For this review, take the finished solid that the model builds, in its own axes (mm). A direction names the side the tool comes from. Coordinates: 2 decimals unless noted, no trailing zeros. Loops run counter-clockwise (first coordinate to the right, second up) from the corner with the lowest first, then second, coordinate; pieces in that order, holes last. Notation, with made-up numbers: M 22.25,81 L 56.25,81 A16 ccw 56.25,100 Z; hole C 23,23.25 d11. An arc over 180 degrees is marked long. Use one line per item in the form item = value.
Autodesk Inventor part; units mm, degrees
ref_plane "YZ Plane" through (0, 0, 0) normal (1, 0, 0) x (0, 1, 0)
ref_plane "XZ Plane" through (0, 0, 0) normal (0, 1, 0) x (-1, 0, 0)
ref_plane "XY Plane" through (0, 0, 0) normal (0, 0, 1) x (1, 0, 0)
sketch "Sketch1" plane through (0, 0, 0) normal (0, 0, 1) x (1, 0, 0)
  arc A0 (18.3475, -1.5748) -> (17.9494, -4.1148) centre (0, 0) ccw
  line L0 (-16.7386, -24.5618) -> (16.7386, -24.5618)
  line L1 (16.7386, -24.5618) -> (16.7386, -12.6068)
  line L2 (-16.7386, -12.6068) -> (-16.7386, -24.5618)
  line L3 (-20.955, 0) -> (-20.955, 20.955) construction
  line L4 (-20.955, 20.955) -> (25.273, 20.955) construction
  line L5 (16.7386, -24.5618) -> (25.273, -24.5618) construction
  line L6 (25.273, -24.5618) -> (25.273, -9.9568) construction
  line L7 (25.273, -9.9568) -> (21.0058, -9.9568) construction
  line L8 (25.273, -9.9568) -> (25.273, 2.1082) construction
  line L9 (25.273, 2.1082) -> (16.2735, 13.2017)
  line L10 (25.273, 2.1082) -> (25.273, -1.5748) construction
  line L11 (25.273, -1.5748) -> (18.3475, -1.5748)
  line L12 (25.273, 2.1082) -> (25.273, -1.5748)
  line L13 (25.273, -1.5748) -> (25.273, -4.1148) construction
  line L14 (25.273, -4.1148) -> (25.273, -9.9568)
  line L15 (25.273, -9.9568) -> (18.4384, -9.9568)
  line L16 (25.273, -4.1148) -> (17.9494, -4.1148)
  arc A1 (16.2735, 13.2017) -> (-16.7386, -12.6068) centre (0, 0) ccw
  arc A2 (16.7386, -12.6068) -> (18.4384, -9.9568) centre (0, 0) ccw
  dimension "d0" = 36.83
extrude "Extrusion1" add sketch "Sketch1" along normal blind 9.525
sketch "Sketch2" plane through (-16.7386, -24.5618, 0) normal (0, -1, 0) x (1, 0, 0)
  line L0 (0, 9.525) -> (33.4772, 9.525)
  line L1 (16.7386, 0) -> (16.7386, 9.525) construction
  line L2 (30.2133, 4.7625) -> (3.2639, 4.7625) construction
  circle A0 centre (3.2639, 4.7625) radius 1.7526
  circle A1 centre (30.2133, 4.7625) radius 1.7526
  dimension "d12" = 26.9494
  dimension "d13" = 3.5052
  dimension "d14" = 3.5052
extrude "Extrusion2" cut sketch "Sketch2" against normal blind 9.525
thread "Thread1"
thread "Thread2"
sketch "Sketch3" plane through (18.4384, -9.9568, 0) normal (0, -1, 0) x (1, 0, 0)
  line L0 (6.8346, 0) -> (6.8346, 9.525)
  line L1 (0, 0) -> (0, 9.525)
  line L2 (6.8346, 4.7625) -> (3.6596, 4.7625) construction
  circle A0 centre (3.6596, 4.7625) radius 1.7526
  point P0 (-18.4384, 0)
  dimension "d21" = 3.175
  dimension "d22" = 3.5052
extrude "Extrusion3" cut sketch "Sketch3" against normal blind 25.4
sketch "Sketch4" plane through (25.273, -1.5748, 0) normal (1, 0, 0) x (0, 0, -1)
  line L0 (0, 3.683) -> (-9.525, 3.683)
  line L1 (-1.8415, 3.683) -> (-7.6835, 3.683)
  line L2 (-7.6835, 3.683) -> (-7.6835, 13.843)
  line L3 (-7.6835, 13.843) -> (-1.8415, 13.843)
  line L4 (-1.8415, 13.843) -> (-1.8415, 3.683)
  point P0 (0, 1.5748)
  dimension "d26" = 10.16
  dimension "d27" = 5.842
extrude "Extrusion4" cut sketch "Sketch4" against normal blind 3.175
sketch "Sketch5" plane through (25.273, 2.1082, 7.6835) normal (0, 1, 0) x (1, 0, 0)
  arc A0 (-3.175, 1.1684) -> (-3.175, 4.6736) centre (-3.175, 2.921) ccw
  circle A1 centre (-3.175, 2.921) radius 2.921
  point P0 (-25.273, 7.6835)
extrude "Extrusion5" cut sketch "Sketch5" along normal blind 9.525
thread "Thread3"
properties part number "Motor Mount"
1. Consider section D-D on y = -20. Write out the cut boundary in (x, z) (1 decimal).
Computed values:
outline = M -16.7,0 L 16.7,0 L 16.7,9.5 L -16.7,9.5 Z; hole C -13.5,4.8 d3.5; hole C 13.5,4.8 d3.5
2. For pin 1 Ø1.1 at (x, z) = (-14, 4.5) entering from -Y; pin 2 Ø4.5 at (x, z) = (22.1, 4.76) entering from +Y; pin 3 Ø5 at (x, z) = (20.5, 5) entering from +Y, all flat-tipped, find the tip position at first contact; note any pin that passes through.
Computed values:
pin_1 = -15.04
pin_2 = 2.11
pin_3 = 11.07
3. Consider section A-A on y = -6. Write out the cut boundary in (x, z) (1 decimal).
Computed values:
outline = M -20.1,0 L -17.4,0 L -17.4,9.5 L -20.1,9.5 Z; M 17.4,0 L 25.3,0 L 25.3,9.5 L 17.4,9.5 Z; hole C 22.1,4.8 d3.5
4. Wall thickness on line 1 along X through (y, z) = (-9.5, 5.75); line 2 along X through (y, z) = (12.5, 3); line 3 along X through (y, z) = (13, 3): over which ranges is each line inside the solid? List them lowest first. Write a range as from..to.
Computed values:
line_1 = -18.68..-15.78, 15.78..20.65, 23.55..25.27
line_2 = -16.82..-13.52, 13.52..16.84
line_3 = -16.44..-13.04, 13.04..16.44
5. Draft analysis for pull direction X (two halves, no side actions). For faces 1 (the face through (13, -15.037, 5)), 2 (the face through (-13.262, 16.224, 4.696)), 3 (the face through (20, -9.957, 6)), 4 (the face through (25.273, -7, 5)), state which applies: +X half, -X half, draft (parallel to the pull), parting line (faces both ways), or undercut.
Computed values:
face_1 = undercut
face_2 = parting line
face_3 = draft
face_4 = +X half
6. Consider section B-B on x = 1. Write out the cut boundary in (y, z) (3 decimals).
Computed values:
outline = M -24.562,0 L -18.388,0 L -18.388,9.525 L -24.562,9.525 Z; M 18.387,0 L 20.931,0 L 20.931,9.525 L 18.387,9.525 Z
7. Tool access review of faces 5 (the face through (12.08, -19.87, 3.7)), 6 (the face through (16.739, -19, 5)), 7 (the face through (20, -4.115, 5)), 8 (the face through (19.178, 4.983, 4.827)), 9 (the face through (-16.739, -19, 5)): name each direction out of +Z, -Z, +X, -X, +Y, -Y from which nothing blocks a thin tool from reaching the whole face with its end or side.
Computed values:
face_5 = -Y
face_6 = +Z, -Z, +X, -Y
face_7 = +Z, -Z, +X
face_8 = +X, +Y
face_9 = +Z, -Z, -X, -Y
8. Consider section C-C on y = 15.5. Write out the cut boundary in (x, z) (3 decimals), plus the area to 3 significant figures.
Computed values:
outline = M -14.102,0 L -9.942,0 L -9.942,9.525 L -14.102,9.525 Z; M 9.942,0 L 14.102,0 L 14.102,9.525 L 9.942,9.525 Z
area = 79.2 mm2
